Can you work these out from the model? Positions are in its coordinate system, mm. A direction names the side the tool comes from. Give positions to 0.01 mm unless a question says otherwise; leave off trailing zeros. Order: outer loops, then holes, each group sorted by start corner. A loop starts at its lowest first (then second) coordinate and runs counter-clockwise, first axis right, second up. Notation, with made-up numbers: (46.25, 58) - (92.25, 58) arc R26 ccw to (92.25, 79) - close; hole circle Ø1 at (0, 44.5). An arc over 180 degrees is marked (long way). One line per question, with ' | ' between items.
```python
from build123d import *

# Parameters (mm, degrees)
SKETCH2_R                        = 30.1625
SKETCH2_R_2                      = 23.8125
BOSS_EXTRUDE1_DEPTH              = 12.7
SKETCH4_R                        = 28.448
SKETCH4_R_2                      = 25.4
CUT_EXTRUDE1_DEPTH               = 2.032
F_1_8_0_125_DIAMETER_HOLE1_D     = 3.175
F_1_8_0_125_DIAMETER_HOLE1_DEPTH = 6.35
F_1_8_0_125_DIAMETER_HOLE1_TIP   = 0.953866233
F_1_8_0_125_DIAMETER_HOLE2_D     = 3.175
F_1_8_0_125_DIAMETER_HOLE2_DEPTH = 6.35
F_1_8_0_125_DIAMETER_HOLE2_TIP   = 0.953866233


with BuildPart() as part:
    # Sketch1 → Revolve1 (revolve)
    with BuildSketch(Plane.XY):
        Polygon((-9.525, -6.35), (-9.525, 0), (-44.45, 0), (-44.45, -20.6375), (-36.3855, -20.6375), (-36.3855, -18.6055), (-33.3375, -18.6055), (-33.3375, -20.6375), (-31.75, -20.6375), (-31.75, -19.05), (-15.875, -6.35), align=None)
    revolve(axis=Axis((0, 0, 0), (0, 1, 0)))

    # Sketch2 → Boss-Extrude1 (add)
    with BuildSketch(Plane(origin=(0, 0, 0), x_dir=(1, 0, 0), z_dir=(0, 1, 0))):
        with Locations((-14.2875, 0)):
            Circle(SKETCH2_R)
        with Locations((-14.2875, 0)):
            Circle(SKETCH2_R_2, mode=Mode.SUBTRACT)
    extrude(amount=BOSS_EXTRUDE1_DEPTH)

    # Sketch4 → Cut-Extrude1 (cut)
    with BuildSketch(Plane(origin=(0, 12.7, 0), x_dir=(1, 0, 0), z_dir=(0, 1, 0))):
        with Locations((-14.2875, 0)):
            Circle(SKETCH4_R)
        with Locations((-14.2875, 0)):
            Circle(SKETCH4_R_2, mode=Mode.SUBTRACT)
    extrude(amount=-CUT_EXTRUDE1_DEPTH, mode=Mode.SUBTRACT)

    # 1/8 (0.125) Diameter Hole1
    with Locations(Plane(origin=(0, -20.6375, 0), x_dir=(-1, 0, 0), z_dir=(0, -1, 0))):
        with Locations((-41.275, 0)):
            Hole(F_1_8_0_125_DIAMETER_HOLE1_D / 2, depth=F_1_8_0_125_DIAMETER_HOLE1_DEPTH)
            with Locations((0, 0, -(F_1_8_0_125_DIAMETER_HOLE1_DEPTH + F_1_8_0_125_DIAMETER_HOLE1_TIP / 2))):  # 118° drill point
                Cone(0, F_1_8_0_125_DIAMETER_HOLE1_D / 2, F_1_8_0_125_DIAMETER_HOLE1_TIP, mode=Mode.SUBTRACT)

    # 1/8 (0.125) Diameter Hole2
    with Locations(Plane(origin=(0, 0, 0), x_dir=(1, 0, 0), z_dir=(0, 1, 0))):
        with Locations((35.745198541, 20.6375)):
            Hole(F_1_8_0_125_DIAMETER_HOLE2_D / 2, depth=F_1_8_0_125_DIAMETER_HOLE2_DEPTH)
            with Locations((0, 0, -(F_1_8_0_125_DIAMETER_HOLE2_DEPTH + F_1_8_0_125_DIAMETER_HOLE2_TIP / 2))):  # 118° drill point
                Cone(0, F_1_8_0_125_DIAMETER_HOLE2_D / 2, F_1_8_0_125_DIAMETER_HOLE2_TIP, mode=Mode.SUBTRACT)


solid = part.part
```
(1) If we mould it in two halves opening along Z, with no side actions, what happens to faces 4 (the face through (41.55, -13.5, -0.01)), 5 (the face through (19, 0, 1)), 6 (the face through (-44.42, 6.26, -1.33))? For each: released by +Z, released by -Z, zero draft, split by the parting line, or undercut.
Answer below:
face 4: undercut | face 5: zero draft | face 6: split by the parting line
(2) On a 3-axis mill with a long thin cutter (end or side, diameter ignored), from which of +Z, -Z, +X, -X, +Y, -Y can I reach the whole of each face in a straight line? I mean faces 1 (the face through (3.5, -20.638, 36.4)), 2 (the face through (-16, -18.606, -29.5)), 3 (the face through (37.33, -3.22, -20.71)). Say none if no direction works.
Answer below:
face 1: +Z, -Z, +X, -X, -Y | face 2: -Y | face 3: +Y
(3) If I drill on line 1 (Z direction, x = 0, y = -19.05); line 2 (X direction, y = -15, z = -0.5); line 3 (X direction, y = 1, z = -1), over which ranges is the centre line in solid material (lowest first)?
Answer below:
line 1: -44.45 to -36.39, -33.34 to -31.75, 31.75 to 33.34, 36.39 to 44.45 | line 2: -44.45 to -26.68, 26.68 to 39.77, 42.78 to 44.45 | line 3: -44.43 to -38.08, 9.5 to 15.86
(4) Will these pins go through, and if not, where does the flat tip stop? pin 1 (25 mm diameter, centred on x = 0, z = 0, fed in from -Y); pin 2 (22 mm diameter, centred on x = -18, z = 16.5, fed in from -Y); pin 3 (3 mm diameter, centred on x = 35.75, z = -20.64, fed in from +Y); pin 4 (10 mm diameter, centred on x = 8.5, y = -12.5, fed in from +Z).
Answer below:
pin 1: y = -6.35 | pin 2: y = -20.64 | pin 3: y = -6.4 | pin 4: z = 44.31
(5) Imagine slicing it at B-B (y = 5). List the corners of the cut face in (x, z) for me (1 decimal), and give its area (3 significant figures).
Answer below:
outline: circle Ø60.3 at (-14.3, 0); hole circle Ø47.6 at (-14.3, 0) | area: 1,080 mm^2
(6) Imagine slicing it at A-A (y = -1.5). Count the separate pieces of the cut face and the enclosed holes in it, and give its area (3 significant figures).
Answer below:
separate pieces: 1 | enclosed holes: 2 | area: 5,910 mm^2
